Verification items for this drawing (mm, ordinates from the low corner). Round coordinates to 2 decimals unless told otherwise and drop trailing zeros. Order: outer loops, then holes, each group sorted by start corner. A loop starts at its lowest first (then second) coordinate and runs counter-clockwise, first axis right, second up. Notation, with made-up numbers: (37, -27) -> (54, -27) arc R29 ccw to (54, 5) -> close; hole circle Ø3 at (-33, 72). An arc over 180 degrees is marked (long way). Answer in a Markdown table with one row per item.
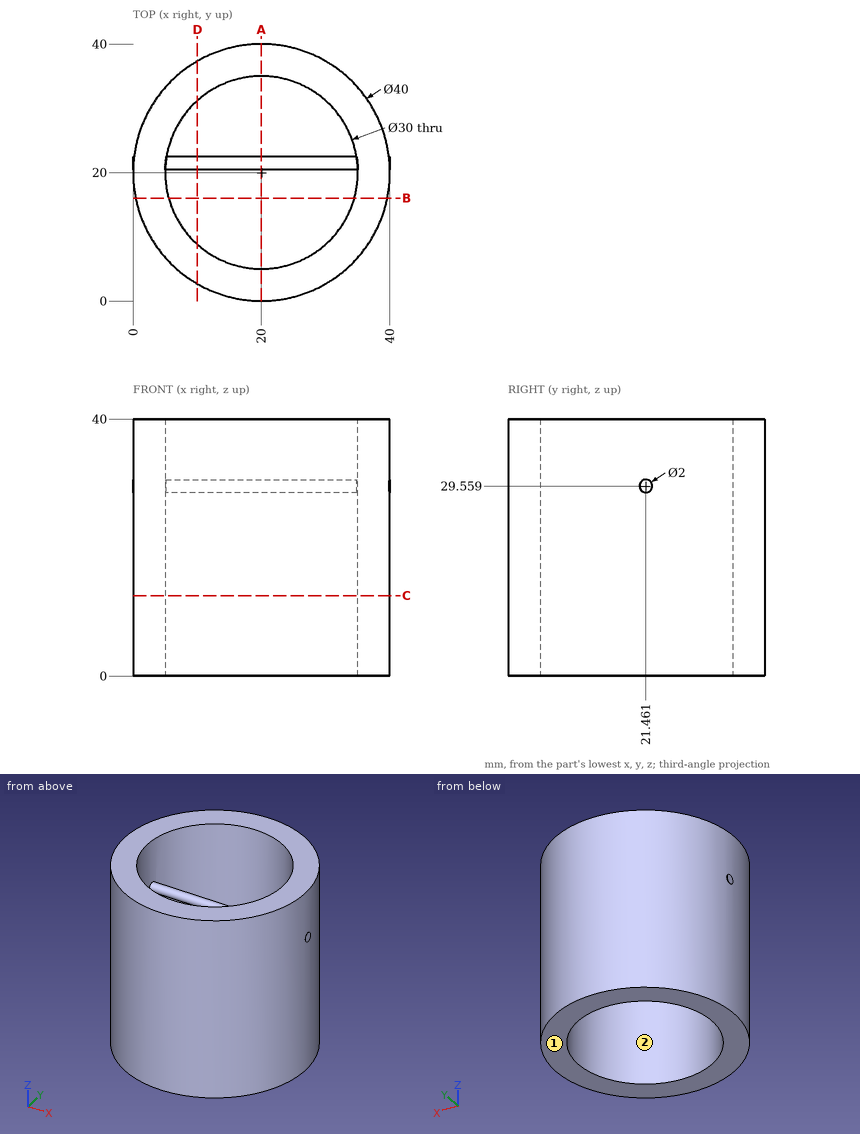
Item 1: Scan lines: line 1 (Y direction, x = 20, z = 18); line 2 (Y direction, x = 22, z = 12.5); line 3 (X direction, y = 25.5, z = 15) (1 decimal). Record each from-to range of solid material in increasing order. Write a range as [from, to].
Result sheet:
| item | result |
|---|---|
| line 1 | y = [0, 5], [35, 40] |
| line 2 | y = [0.1, 5.13], [34.87, 39.9] |
| line 3 | x = [0.8, 6], [34, 39.2] |
Item 2: Cross-section at B-B (y = 16). Record the boundary of the cut face in (x, z).
Result sheet:
| item | result |
|---|---|
| outline | (0.4, 0) -> (5.54, 0) -> (5.54, 40) -> (0.4, 40) -> close; (34.46, 0) -> (39.6, 0) -> (39.6, 40) -> (34.46, 40) -> close |
Item 3: Cross-section at C-C (z = 12.5). Record the boundary of the cut face in (x, y).
Result sheet:
| item | result |
|---|---|
| outline | circle Ø40 at (20, 20); hole circle Ø30 at (20, 20) |
Item 4: Mould release check, pull along Y, two halves, no side actions. Record for the marked faces 1 and 2: pulls with the +Y half, pulls with the -Y half, needs draft (parallel to the pull), parting line crosses it, or undercut.
Result sheet:
| item | result |
|---|---|
| face 1 | needs draft |
| face 2 | undercut |
Item 5: Depth check by flat-ended pin: P1, Ø4, axis at y = 9, z = 27, coming from the +X side; P2, Ø2, axis at y = 5.5, z = 13, coming from the +X side; P3, Ø8, axis at x = 16.5, z = 8.5, coming from the -Y side. Enter the tip coordinate at first touch or a pass-through.
Result sheet:
| item | result |
|---|---|
| P1 | stops at x = 37.86 |
| P2 | stops at x = 34.76 |
| P3 | stops at y = 0 |
Item 6: Cross-section at A-A (x = 20). Record the boundary of the cut face in (y, z), and give its area (3 significant figures).
Result sheet:
| item | result |
|---|---|
| outline | (0, 0) -> (5, 0) -> (5, 40) -> (0, 40) -> close; circle Ø2 at (21.46, 29.56); (35, 0) -> (40, 0) -> (40, 40) -> (35, 40) -> close |
| area | 403 mm^2 |
Item 7: Cross-section at D-D (x = 10). Record the boundary of the cut face in (y, z), and give its area (3 significant figures).
Result sheet:
| item | result |
|---|---|
| outline | (2.68, 0) -> (8.82, 0) -> (8.82, 40) -> (2.68, 40) -> close; circle Ø2 at (21.46, 29.56); (31.18, 0) -> (37.32, 0) -> (37.32, 40) -> (31.18, 40) -> close |
| area | 494 mm^2 |
